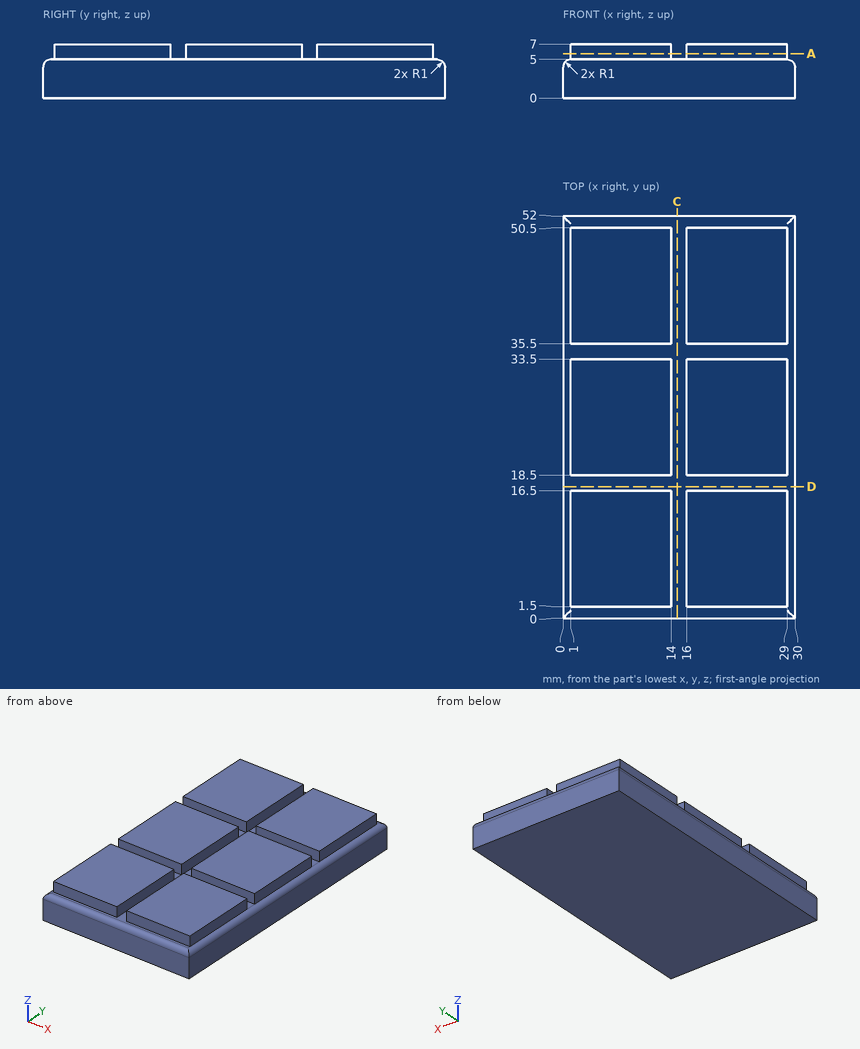
Input: dimensioned drawing with shaded views. Units: mm. Origin: part minimum x, y, z. Give positions to 0.01 mm unless a question says otherwise; leave off trailing zeros. Write each loop counter-clockwise with the first axis right and the second up, starting at its lowest first coordinate (ties: lowest second). Pieces come first, ordered by that corner, then holes. Notation, with made-up numbers: (14.25, 33.5) -> (48.25, 33.5) arc R19 ccw to (48.25, 63.5) -> close; hole circle Ø11 at (54, -7). An arc over 180 degrees is marked (long way). Answer as a JSON object with one key per item and string values.
1. Cut plane D-D on y = 17. Output: boundary loops of the cut face in (x, z), and give its area (3 significant figures).
Ans:
{"outline": "(0, 0) -> (30, 0) -> (30, 4) arc R1 ccw to (29, 5) -> (1, 5) arc R1 ccw to (0, 4) -> close", "area": "150 mm^2"}
2. Ray query, probe 1 along Y at (x, z) = (9.5, 5.25); probe 2 along X at (y, z) = (33, 6.5); probe 3 along Z at (x, y) = (14.5, 26.5). Return the intervals inside material, ascending. Write a range as from..to.
Ans:
{"probe 1": "y = 1.5..16.5, 18.5..33.5, 35.5..50.5", "probe 2": "x = 1..14, 16..29", "probe 3": "z = 0..5"}
3. Cut plane A-A on z = 5.75. Output: boundary loops of the cut face in (x, y).
Ans:
{"outline": "(1, 1.5) -> (14, 1.5) -> (14, 16.5) -> (1, 16.5) -> close; (1, 18.5) -> (14, 18.5) -> (14, 33.5) -> (1, 33.5) -> close; (1, 35.5) -> (14, 35.5) -> (14, 50.5) -> (1, 50.5) -> close; (16, 1.5) -> (29, 1.5) -> (29, 16.5) -> (16, 16.5) -> close; (16, 18.5) -> (29, 18.5) -> (29, 33.5) -> (16, 33.5) -> close; (16, 35.5) -> (29, 35.5) -> (29, 50.5) -> (16, 50.5) -> close"}
4. Cut plane C-C on x = 14.75. Output: boundary loops of the cut face in (y, z), and give its area (3 significant figures).
Ans:
{"outline": "(0, 0) -> (52, 0) -> (52, 4) arc R1 ccw to (51, 5) -> (1, 5) arc R1 ccw to (0, 4) -> close", "area": "260 mm^2"}
5. Contact query for flat-ended pins moving along their axis: pin 1 (0.6 mm diameter, centred on y = 43.5, z = 6.5, fed in from +X); pin 2 (2 mm diameter, centred on y = 32.5, z = 5.5, fed in from -X); pin 3 (1 mm diameter, centred on y = 28, z = 6.5, fed in from -X). Output: stop coordinate, or through.
Ans:
{"pin 1": "stops at x = 29", "pin 2": "stops at x = 0.13", "pin 3": "stops at x = 1"}
